Check sheet for the modelled part. Datum: model origin and axes. Units: mm. A direction names the side the tool comes from. Coordinates: 2 decimals unless noted, no trailing zeros. Write each loop counter-clockwise with the first axis right and the second up, starting at its lowest first coordinate (ties: lowest second). Pieces come first, ordered by that corner, then holes. Notation, with made-up numbers: (68.25, 70.25) -> (90.25, 70.25) arc R20 ccw to (90.25, 107.25) -> close; hole circle Ø2 at (85, -7.75). An arc over 180 degrees is marked (long way). One line per item, written item: value. Start each with the question number.
1) Gauge pin test, flat ends, axial feed: P1, Ø3.5, axis at x = -26.25, y = 59, coming from the +Z side; P2, Ø7, axis at x = 90.5, y = -1.8, coming from the +Z side; P3, Ø3, axis at x = 25, z = 6, coming from the -Y side. Record the tip position at first contact, or that the pin passes through.
2) Scan lines: line 1 along Y through (x, z) = (-68.25, 0.6); line 2 along Y through (x, z) = (-36.75, 0.9); line 3 along Y through (x, z) = (-90.5, 1.15). Record each from-to range of solid material in increasing order. Write a range as [from, to].
3) Draft check along X on faces 3 (the cylindrical face through (-98.584, 66.441, 8.381)), 4 (the flat face through (105.3, 9.4, 9.4)), 5 (the cylindrical face through (96.847, -45.766, 0.986)). Enter one of: +X half, -X half, draft (parallel to the pull), parting line (faces both ways), or undercut.
4) Sectioned sample at A-A on x = 26.25. Enter the section's corners in (y, z), plus the area to 3 significant figures.
5) Sectioned sample at D-D on y = 59. Give the number of separate pieces and of enclosed holes in the cut face, plus the area to 3 significant figures.
6) Sectioned sample at B-B on y = 29.7. Enter the section's corners in (x, z), plus the area to 3 significant figures.
7) Set-up check for faces 1 (the cylindrical face through (-35.753, 57.084, 0.986)), 2 (the flat face through (-1, 50, 2)): record each of +Z, -Z, +X, -X, +Y, -Y from which the full face is reachable in a straight line by a thin tool's end or side.
8) Sectioned sample at C-C on x = -22. Enter the section's corners in (y, z).
```python
from build123d import *

# Parameters (mm, degrees)
PAD001_DEPTH      = 15
FILLET_R          = 1.5
SKETCH002_R       = 2.16
SKETCH002_R_2     = 2
SKETCH002_W       = 150
SKETCH002_H       = 88.7
PAD_DEPTH         = 2
CHAMFER_SIZE      = 1.8
PAD002_DEPTH      = 150
PAD002_DEPTH_BACK = 150
FILLET001_R       = 1.5
FILLET002_R       = 1.5
FILLET003_R       = 1.5


with BuildPart() as hat:
    # Sketch003 → Pad001 (new body)
    with BuildSketch(Plane.XY):
        with BuildLine():
            Line((-105.5, -52), (105.5, -52))
            Line((105.5, -52), (105.5, 50))
            ThreePointArc((105.5, 50), (98.763456, 66.263456), (82.5, 73))
            Line((-82.5, 73), (82.5, 73))
            ThreePointArc((-82.5, 73), (-98.763456, 66.263456), (-105.5, 50))
            Line((-105.5, -52), (-105.5, 50))
        make_face()
        with BuildLine():
            Line((-103.5, -50), (103.5, -50))
            Line((103.5, -50), (103.5, 50))
            ThreePointArc((103.5, 50), (97.349242, 64.849242), (82.5, 71))
            Line((-82.5, 71), (82.5, 71))
            ThreePointArc((-82.5, 71), (-97.349242, 64.849242), (-103.5, 50))
            Line((-103.5, -50), (-103.5, 50))
        make_face(mode=Mode.SUBTRACT)
    extrude(amount=PAD001_DEPTH)

    # Fillet
    fillet_edges = [hat.edges().sort_by_distance(p)[0] for p in [
        (0, 71, 15),
    ]]
    fillet(fillet_edges, radius=FILLET_R)


with BuildPart() as hat_1:
    # Body001 placement: moved
    add(hat.part.moved(Location((0, 0, 2))))


with BuildPart() as front:
    # Sketch002 → Pad (new body)
    with BuildSketch(Plane.XY):
        with BuildLine():
            Line((-105.5, -52), (105.5, -52))
            Line((105.5, -52), (105.5, 50))
            ThreePointArc((105.5, 50), (98.763456, 66.263456), (82.5, 73))
            Line((-82.5, 73), (82.5, 73))
            ThreePointArc((-82.5, 73), (-98.763456, 66.263456), (-105.5, 50))
            Line((-105.5, -52), (-105.5, 50))
        make_face()
        with Locations((-90.5, 40.2)):
            Circle(SKETCH002_R, mode=Mode.SUBTRACT)
        with Locations((90.5, 40.2)):
            Circle(SKETCH002_R, mode=Mode.SUBTRACT)
        with Locations((-68.25, 59)):
            Circle(SKETCH002_R, mode=Mode.SUBTRACT)
        with Locations((-57.75, 59)):
            Circle(SKETCH002_R, mode=Mode.SUBTRACT)
        with Locations((-47.25, 59)):
            Circle(SKETCH002_R, mode=Mode.SUBTRACT)
        with Locations((-36.75, 59)):
            Circle(SKETCH002_R, mode=Mode.SUBTRACT)
        with Locations((-26.25, 59)):
            Circle(SKETCH002_R, mode=Mode.SUBTRACT)
        with Locations((-15.75, 59)):
            Circle(SKETCH002_R, mode=Mode.SUBTRACT)
        with Locations((-5.25, 59)):
            Circle(SKETCH002_R, mode=Mode.SUBTRACT)
        with Locations((5.25, 59)):
            Circle(SKETCH002_R, mode=Mode.SUBTRACT)
        with Locations((15.75, 59)):
            Circle(SKETCH002_R, mode=Mode.SUBTRACT)
        with Locations((26.25, 59)):
            Circle(SKETCH002_R, mode=Mode.SUBTRACT)
        with Locations((36.75, 59)):
            Circle(SKETCH002_R, mode=Mode.SUBTRACT)
        with Locations((47.25, 59)):
            Circle(SKETCH002_R, mode=Mode.SUBTRACT)
        with Locations((57.75, 59)):
            Circle(SKETCH002_R, mode=Mode.SUBTRACT)
        with Locations((68.25, 59)):
            Circle(SKETCH002_R, mode=Mode.SUBTRACT)
        with Locations((-90.5, 29.7)):
            Circle(SKETCH002_R, mode=Mode.SUBTRACT)
        with Locations((-90.5, 19.2)):
            Circle(SKETCH002_R, mode=Mode.SUBTRACT)
        with Locations((-90.5, 8.7)):
            Circle(SKETCH002_R, mode=Mode.SUBTRACT)
        with Locations((-90.5, -1.8)):
            Circle(SKETCH002_R, mode=Mode.SUBTRACT)
        with Locations((90.5, 29.7)):
            Circle(SKETCH002_R, mode=Mode.SUBTRACT)
        with Locations((90.5, 19.2)):
            Circle(SKETCH002_R, mode=Mode.SUBTRACT)
        with Locations((90.5, 8.7)):
            Circle(SKETCH002_R, mode=Mode.SUBTRACT)
        with Locations((90.5, -1.8)):
            Circle(SKETCH002_R, mode=Mode.SUBTRACT)
        with Locations((-95, -45)):
            Circle(SKETCH002_R_2, mode=Mode.SUBTRACT)
        with Locations((95, -45)):
            Circle(SKETCH002_R_2, mode=Mode.SUBTRACT)
        with Locations((95, 55)):
            Circle(SKETCH002_R_2, mode=Mode.SUBTRACT)
        with Locations((-95, 55)):
            Circle(SKETCH002_R_2, mode=Mode.SUBTRACT)
        with Locations((0, 1.85)):
            Rectangle(SKETCH002_W, SKETCH002_H, mode=Mode.SUBTRACT)
    extrude(amount=PAD_DEPTH)

    # Chamfer
    chamfer_edges = [front.edges().sort_by_distance(p)[0] for p in [
        (0, 46.2, 2),
        (-75, 1.85, 2),
        (75, 1.85, 2),
        (0, -42.5, 2),
    ]]
    chamfer(chamfer_edges, length=CHAMFER_SIZE)


with BuildPart() as top:
    # Sketch004 → Pad002 (new body, two sides)
    with BuildSketch(Plane.YZ) as pad002_sk:
        Polygon((0, 0), (28.284271, 28.284271), (88.284271, 28.284271), (88.284271, 0), align=None)
    extrude(amount=PAD002_DEPTH)
    extrude(pad002_sk.sketch, amount=-PAD002_DEPTH_BACK)

    # Boolean: intersect HAT
    add(hat_1.part, mode=Mode.INTERSECT)

    # Fillet001
    fillet001_edges = [top.edges().sort_by_distance(p)[0] for p in [
        (-103.5, 8.75, 8.75),
    ]]
    fillet(fillet001_edges, radius=FILLET001_R)

    # Fillet002
    fillet002_edges = [top.edges().sort_by_distance(p)[0] for p in [
        (103.5, 8.75, 8.75),
    ]]
    fillet(fillet002_edges, radius=FILLET002_R)

    # Boolean001: union FRONT
    add(front.part)

    # Fillet003
    fillet003_edges = [top.edges().sort_by_distance(p)[0] for p in [
        (-103.5, 27.06066, 2),
    ]]
    fillet(fillet003_edges, radius=FILLET003_R)


solid = top.part
```
Answers:
1. P1: passes through
1. P2: stops at z = 2
1. P3: stops at y = 71
2. line 1: y = [-52, -42.9], [46.6, 56.84], [61.16, 73]
2. line 2: y = [-52, -43.2], [46.9, 56.84], [61.16, 73]
2. line 3: y = [-52, -3.96], [0.36, 6.54], [10.86, 17.04], [21.36, 27.54], [31.86, 38.04], [42.36, 71.56]
3. face 3: -X half
3. face 4: draft
3. face 5: undercut
4. outline: (-52, 0) -> (-42.5, 0) -> (-42.5, 0.2) -> (-44.3, 2) -> (-52, 2) -> close; (46.2, 0) -> (56.84, 0) -> (56.84, 2) -> (48, 2) -> (46.2, 0.2) -> close; (61.16, 0) -> (73, 0) -> (73, 17) -> (72.5, 17) arc R1.5 ccw to (71, 15.5) -> (71, 3.5) arc R1.5 cw to (69.5, 2) -> (61.16, 2) -> close
4. area: 90.7 mm2
5. separate pieces: 15
5. enclosed holes: 0
5. area: 359 mm2
6. outline: (-105.5, 0) -> (-92.66, 0) -> (-92.66, 2) -> (-102, 2) arc R1.5 cw to (-103.5, 3.5) -> (-103.5, 15.5) arc R1.5 ccw to (-105, 17) -> (-105.5, 17) -> close; (-88.34, 0) -> (-75, 0) -> (-75, 0.2) -> (-76.8, 2) -> (-88.34, 2) -> close; (75, 0) -> (88.34, 0) -> (88.34, 2) -> (76.8, 2) -> (75, 0.2) -> close; (92.66, 0) -> (105.5, 0) -> (105.5, 17) -> (105, 17) arc R1.5 ccw to (103.5, 15.5) -> (103.5, 3.5) arc R1.5 cw to (102, 2) -> (92.66, 2) -> close
6. area: 161 mm2
7. face 1: +Z, -Z
7. face 2: +Z, -Y
8. outline: (-52, 0) -> (-42.5, 0) -> (-42.5, 0.2) -> (-44.3, 2) -> (-52, 2) -> close; (46.2, 0) -> (73, 0) -> (73, 17) -> (72.5, 17) arc R1.5 ccw to (71, 15.5) -> (71, 3.5) arc R1.5 cw to (69.5, 2) -> (48, 2) -> (46.2, 0.2) -> close
